```python
from build123d import *

# Parameters (mm, degrees)
F0_R      = 15
F1_DEPTH  = 12
F2_R      = 5
F3_DEPTH  = 10
F4_R      = 12.5
F5_DEPTH  = 2
F5_TAPER  = 45
F6_R      = 10.5
F7_DEPTH  = 2
F7_TAPER  = -45
F8_R      = 10
F9_DEPTH  = 2
F9_TAPER  = 45
F10_R     = 8
F11_DEPTH = 2
F11_TAPER = -45
F12_R     = 14
F13_DEPTH = 2
F13_TAPER = 45
F14_R     = 12
F15_DEPTH = 2
F15_TAPER = -45
F16_R     = 9
F17_DEPTH = 2
F17_TAPER = 45
F18_R     = 7
F19_DEPTH = 2
F19_TAPER = -45
F20_R     = 12.5
F21_DEPTH = 2
F21_TAPER = 45
F22_R     = 10.5
F23_DEPTH = 2
F23_TAPER = -45
F24_R     = 5
F25_DEPTH = 10


with BuildPart() as f1:
    # F0 (on Front) → F1 (new body)
    with BuildSketch(Plane.XZ):
        Circle(F0_R)
    extrude(amount=F1_DEPTH)

    # F2 (on face) → F3 (join)
    with BuildSketch(Plane.XZ.offset(12)):
        Circle(F2_R)
    extrude(amount=F3_DEPTH)

    # F4 (on face) → F5 (join)
    with BuildSketch(Plane.XZ.offset(22)):
        Circle(F4_R)
    extrude(amount=F5_DEPTH, taper=F5_TAPER)

    # F6 (on face) → F7 (join)
    with BuildSketch(Plane.XZ.offset(24)):
        Circle(F6_R)
    extrude(amount=F7_DEPTH, taper=F7_TAPER)

    # F8 (on face) → F9 (join)
    with BuildSketch(Plane.XZ.offset(26)):
        Circle(F8_R)
    extrude(amount=F9_DEPTH, taper=F9_TAPER)

    # F10 (on face) → F11 (join)
    with BuildSketch(Plane.XZ.offset(28)):
        Circle(F10_R)
    extrude(amount=F11_DEPTH, taper=F11_TAPER)

    # F12 (on face) → F13 (join)
    with BuildSketch(Plane.XZ.offset(30)):
        Circle(F12_R)
    extrude(amount=F13_DEPTH, taper=F13_TAPER)

    # F14 (on face) → F15 (join)
    with BuildSketch(Plane.XZ.offset(32)):
        Circle(F14_R)
    extrude(amount=F15_DEPTH, taper=F15_TAPER)

    # F16 (on face) → F17 (join)
    with BuildSketch(Plane.XZ.offset(34)):
        Circle(F16_R)
    extrude(amount=F17_DEPTH, taper=F17_TAPER)

    # F18 (on face) → F19 (join)
    with BuildSketch(Plane.XZ.offset(36)):
        Circle(F18_R)
    extrude(amount=F19_DEPTH, taper=F19_TAPER)

    # F20 (on face) → F21 (join)
    with BuildSketch(Plane.XZ.offset(38)):
        Circle(F20_R)
    extrude(amount=F21_DEPTH, taper=F21_TAPER)

    # F22 (on face) → F23 (join)
    with BuildSketch(Plane.XZ.offset(40)):
        Circle(F22_R)
    extrude(amount=F23_DEPTH, taper=F23_TAPER)

    # F24 (on face) → F25 (join)
    with BuildSketch(Plane.XZ.offset(42)):
        Circle(F24_R)
    extrude(amount=F25_DEPTH)


solid = f1.part
```
Part model, mm, in its own coordinate system. A direction names the side the tool comes from. Coordinates: 2 decimals unless noted, no trailing zeros. Order: outer loops, then holes, each group sorted by start corner. A loop starts at its lowest first (then second) coordinate and runs counter-clockwise, first axis right, second up. Notation, with made-up numbers: (-12.75, -2.75) - (12.25, -2.75) arc R15 ccw to (12.25, 18.25) - close; hole circle Ø8 at (60, 37). An arc over 180 degrees is marked (long way). Return JSON: item names as keys, results as strings. Group by question number.
Item 1: Drill centre lines: probe 1 along Y at (x, z) = (9.75, 3.5); probe 2 along Y at (x, z) = (-5.5, -2.75); probe 3 along Y at (x, z) = (-7.5, -1.5). Where is each one in solid material? Low to high. Write a range as from..to.
Item 2: Pin check, flat tips, straight feed: pin 1 (3 mm diameter, centred on y = -24.5, z = -9, fed in from +X); pin 2 (1 mm diameter, centred on x = -9, y = -31.5, fed in from +Z); pin 3 (8 mm diameter, centred on x = 12, z = -3, fed in from -Y). Stop position of each tip, or through.
Item 3: Which spindle directions (+Z, -Z, +X, -X, +Y, -Y) get a long thin tool onto all of the face, cutting with end or side? Do faces 1 (the face through (-4, -12, 4)), 2 (the face through (0, -52, 0)), 3 (the face through (-1.08, -46.93, -4.88)). Say none if no direction does.
Item 4: Cut at A-A (y = -43). List the corners of the cut face in (x, z), plus the area to 3 significant figures.
Check values:
{
 "1": {"probe 1": "y = -42..-38, -34..-30, -26..-22, -12..0", "probe 2": "y = -42..-22, -12..0", "probe 3": "y = -42..-36.65, -35.35..-22, -12..0"},
 "2": {"pin 1": "stops at x = 9.13", "pin 2": "stops at z = 9.53", "pin 3": "stops at y = -42"},
 "3": {"face 1": "none", "face 2": "+Z, -Z, +X, -X, -Y", "face 3": "-Y"},
 "4": {"outline": "circle Ø10 at (0, 0)", "area": "78.5 mm2"}
}
